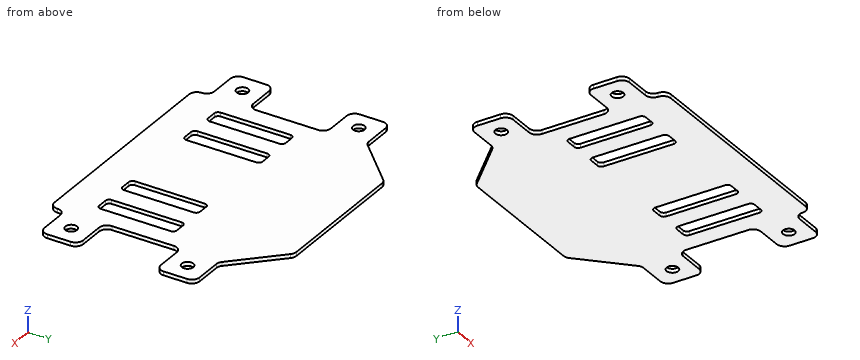
```python
from build123d import *

# Parameters (mm, degrees)
MODEL_R         = 1.5
EXTRUDE_1_DEPTH = 1


with BuildPart() as part:
    # Model → Бобышка-Вытянуть1 (new body)
    with BuildSketch(Plane.XY):
        with BuildLine():
            Line((-29.5, 16), (-29.5, 32))
            ThreePointArc((-29.5, 32), (-30.085786438, 33.414213562), (-31.5, 34))
            Line((-31.5, 34), (-38, 34))
            ThreePointArc((-38, 34), (-39.414213562, 34.585786438), (-40, 36))
            Line((-40, 36), (-40, 42))
            ThreePointArc((-40, 42), (-39.414213562, 43.414213562), (-38, 44))
            Line((-38, 44), (-31.156854249, 44))
            ThreePointArc((-31.156854249, 44), (-30.391487385, 44.152240935), (-29.742640687, 44.585786438))
            Line((-29.742640687, 44.585786438), (-18.914213562, 55.414213562))
            ThreePointArc((-18.914213562, 55.414213562), (-18.265366865, 55.847759065), (-17.5, 56))
            Line((-17.5, 56), (0, 56))
            Line((0, 56), (17.5, 56))
            ThreePointArc((17.5, 56), (18.265366865, 55.847759065), (18.914213562, 55.414213562))
            Line((18.914213562, 55.414213562), (29.742640687, 44.585786438))
            ThreePointArc((29.742640687, 44.585786438), (30.391487385, 44.152240935), (31.156854249, 44))
            Line((31.156854249, 44), (38, 44))
            ThreePointArc((38, 44), (39.414213562, 43.414213562), (40, 42))
            Line((40, 42), (40, 36))
            ThreePointArc((40, 36), (39.414213562, 34.585786438), (38, 34))
            Line((38, 34), (31.5, 34))
            ThreePointArc((31.5, 34), (30.085786438, 33.414213562), (29.5, 32))
            Line((29.5, 32), (29.5, 16))
            ThreePointArc((29.5, 16), (30.085786438, 14.585786438), (31.5, 14))
            Line((31.5, 14), (38, 14))
            ThreePointArc((38, 14), (39.414213562, 13.414213562), (40, 12))
            Line((40, 12), (40, 6))
            ThreePointArc((40, 6), (39.414213562, 4.585786438), (38, 4))
            Line((38, 4), (31.5, 4))
            ThreePointArc((31.5, 4), (30.085786438, 3.414213562), (29.5, 2))
            ThreePointArc((29.5, 2), (28.914213562, 0.585786438), (27.5, 0))
            Line((27.5, 0), (0, 0))
            Line((0, 0), (-27.5, 0))
            ThreePointArc((-27.5, 0), (-28.914213562, 0.585786438), (-29.5, 2))
            ThreePointArc((-29.5, 2), (-30.085786438, 3.414213562), (-31.5, 4))
            Line((-31.5, 4), (-38, 4))
            ThreePointArc((-38, 4), (-39.414213562, 4.585786438), (-40, 6))
            Line((-40, 6), (-40, 12))
            ThreePointArc((-40, 12), (-39.414213562, 13.414213562), (-38, 14))
            Line((-38, 14), (-31.5, 14))
            ThreePointArc((-31.5, 14), (-30.085786438, 14.585786438), (-29.5, 16))
        make_face()
        with Locations((-35, 9)):
            Circle(MODEL_R, mode=Mode.SUBTRACT)
        with Locations((-35, 39)):
            Circle(MODEL_R, mode=Mode.SUBTRACT)
        with Locations((35, 9)):
            Circle(MODEL_R, mode=Mode.SUBTRACT)
        with Locations((35, 39)):
            Circle(MODEL_R, mode=Mode.SUBTRACT)
        with BuildLine():
            Line((-23.5, 9), (-21, 9))
            ThreePointArc((-21, 9), (-20.292893219, 9.292893219), (-20, 10))
            Line((-20, 10), (-20, 28))
            ThreePointArc((-20, 28), (-20.292893219, 28.707106781), (-21, 29))
            Line((-21, 29), (-23.5, 29))
            ThreePointArc((-23.5, 29), (-24.207106781, 28.707106781), (-24.5, 28))
            Line((-24.5, 28), (-24.5, 10))
            ThreePointArc((-24.5, 10), (-24.207106781, 9.292893219), (-23.5, 9))
        make_face(mode=Mode.SUBTRACT)
        with BuildLine():
            Line((-14, 9), (-11.5, 9))
            ThreePointArc((-11.5, 9), (-10.792893219, 9.292893219), (-10.5, 10))
            Line((-10.5, 10), (-10.5, 28))
            ThreePointArc((-10.5, 28), (-10.792893219, 28.707106781), (-11.5, 29))
            Line((-11.5, 29), (-14, 29))
            ThreePointArc((-14, 29), (-14.707106781, 28.707106781), (-15, 28))
            Line((-15, 28), (-15, 10))
            ThreePointArc((-15, 10), (-14.707106781, 9.292893219), (-14, 9))
        make_face(mode=Mode.SUBTRACT)
        with BuildLine():
            Line((23.5, 9), (21, 9))
            ThreePointArc((21, 9), (20.292893219, 9.292893219), (20, 10))
            Line((20, 10), (20, 28))
            ThreePointArc((20, 28), (20.292893219, 28.707106781), (21, 29))
            Line((21, 29), (23.5, 29))
            ThreePointArc((23.5, 29), (24.207106781, 28.707106781), (24.5, 28))
            Line((24.5, 28), (24.5, 10))
            ThreePointArc((24.5, 10), (24.207106781, 9.292893219), (23.5, 9))
        make_face(mode=Mode.SUBTRACT)
        with BuildLine():
            Line((14, 9), (11.5, 9))
            ThreePointArc((11.5, 9), (10.792893219, 9.292893219), (10.5, 10))
            Line((10.5, 10), (10.5, 28))
            ThreePointArc((10.5, 28), (10.792893219, 28.707106781), (11.5, 29))
            Line((11.5, 29), (14, 29))
            ThreePointArc((14, 29), (14.707106781, 28.707106781), (15, 28))
            Line((15, 28), (15, 10))
            ThreePointArc((15, 10), (14.707106781, 9.292893219), (14, 9))
        make_face(mode=Mode.SUBTRACT)
    extrude(amount=EXTRUDE_1_DEPTH)


solid = part.part
```
The model under review builds one solid part; all positions refer to its coordinate system, in mm. Round coordinates to 2 decimals unless told otherwise and drop trailing zeros. Loops run counter-clockwise (first coordinate to the right, second up) from the corner with the lowest first, then second, coordinate; pieces in that order, holes last. Notation, with made-up numbers: M -32,50 L -19,50 A20 ccw -19,74 Z; hole C -16.5,-7 d11. An arc over 180 degrees is marked long. Answer as a JSON object with one key per item and string values.
(1) Clearance check with flat-ended pins moving along their axes: P1, Ø1, axis at x = 7.5, y = 12, coming from the -Z side; P2, Ø0.5, axis at x = 35.5, z = 0.5, coming from the +Y side. State where each tip first meets the part, or that it passes through.
Resolved:
{"P1": "z = 0", "P2": "y = 44"}
(2) Take a section at C-C on z = 0.65. Count the separate pieces of the cut face and the enclosed holes in it, and give its area (3 significant figures).
Resolved:
{"separate pieces": "1", "enclosed holes": "8", "area": "3,210 mm²"}
(3) To check wall thickness, follow line 1 along X through (y, z) = (20, 0.55); line 2 along Y through (x, z) = (35, 0.5); line 3 along Y through (x, z) = (-35.5, 0.8). State the ranges of each line that lie inside material, in increasing order.
Resolved:
{"line 1": "-29.5 to -24.5, -20 to -15, -10.5 to 10.5, 15 to 20, 24.5 to 29.5", "line 2": "4 to 7.5, 10.5 to 14, 34 to 37.5, 40.5 to 44", "line 3": "4 to 7.59, 10.41 to 14, 34 to 37.59, 40.41 to 44"}
(4) Take a section at A-A on x = -35. Give the boundary of the cut face in (y, z).
Resolved:
{"outline": "M 4,0 L 7.5,0 L 7.5,1 L 4,1 Z; M 10.5,0 L 14,0 L 14,1 L 10.5,1 Z; M 34,0 L 37.5,0 L 37.5,1 L 34,1 Z; M 40.5,0 L 44,0 L 44,1 L 40.5,1 Z"}
(5) Take a section at B-B on y = 39. Give the boundary of the cut face in (x, z), and give its area (3 significant figures).
Resolved:
{"outline": "M -40,0 L -36.5,0 L -36.5,1 L -40,1 Z; M -33.5,0 L 33.5,0 L 33.5,1 L -33.5,1 Z; M 36.5,0 L 40,0 L 40,1 L 36.5,1 Z", "area": "74.0 mm²"}
